Autodesk Inventor part; units mm, degrees
ref_plane "YZ Plane" through (0, 0, 0) normal (1, 0, 0) x (0, 1, 0)
ref_plane "XZ Plane" through (0, 0, 0) normal (0, 1, 0) x (-1, 0, 0)
ref_plane "XY Plane" through (0, 0, 0) normal (0, 0, 1) x (1, 0, 0)
sketch "Sketch1" plane through (0, 0, 0) normal (1, 0, 0) x (0, 1, 0)
  circle A0 centre (0, 0) radius 2.25
  circle A1 centre (0, 0) radius 4.75
  line L0 (0, 4.75) -> (-10.16, 4.75)
  line L1 (0, -4.75) -> (-10.16, -4.75)
  line L2 (-10.16, 4.75) -> (-10.16, -4.75)
  dimension "d0" = 4.5
  dimension "d1" = 9.5
  dimension "d2" = 10.16
  dimension "d3" = 10.16
extrude "Extrusion1" add sketch "Sketch1" along normal blind 7.62
ref_plane "Work Plane1" through (15.24, 0, 0) normal (1, 0, 0) x (0, 0, -1)
mirror "Mirror1" about plane through (15.24, 0, 0) normal (1, 0, 0) of "Extrusion1"
sketch "Sketch2" plane through (30.48, -10.16, 4.75) normal (1, 0, 0) x (0, 0, -1)
  circle A0 centre (4.75, 10.16) radius 2.25
  line L0 (7.5, 8.5723) -> (4.75, 6.9846)
  line L1 (4.75, 6.9846) -> (2, 8.5723)
  line L2 (2, 8.5723) -> (2, 11.7477)
  line L3 (2, 11.7477) -> (4.75, 13.3354)
  line L4 (4.75, 13.3354) -> (7.5, 11.7477)
  line L5 (7.5, 11.7477) -> (7.5, 8.5723)
  dimension "d7" = 5.5
extrude "Extrusion2" cut sketch "Sketch2" against normal blind 1.5
sketch "Sketch3" plane through (0, 0, 0) normal (-1, 0, 0) x (0, 0, 1)
  circle A0 centre (0, 0) radius 2.75
  dimension "d10" = 5.5
extrude "Extrusion3" cut sketch "Sketch3" against normal blind 1.5
sketch "Sketch4" plane through (0, 0, 0) normal (-1, 0, 0) x (0, 0, 1)
  line L0 (4.75, 0) -> (7.925, -10.16)
  line L1 (4.75, -10.16) -> (-4.75, -10.16)
  line L2 (7.925, -10.16) -> (4.75, -10.16)
  line L3 (4.75, 0) -> (4.75, -10.16)
  point P0 (0, 0)
  dimension "d13" = 3.175
extrude "Extrusion4" add sketch "Sketch4" against normal up to surface (30.48 mm away)
sketch "Sketch5" plane through (0, 0, 0) normal (-1, 0, 0) x (0, 0, 1)
  line L0 (-4.75, -10.16) -> (-4.75, 0)
  line L1 (-4.75, -10.16) -> (-4.75, -31.75)
  line L2 (4.75, 0) -> (4.75, -10.16)
  line L3 (7.925, -10.16) -> (14.6719, -31.75)
  line L4 (4.75, 0) -> (7.925, -10.16)
  line L5 (-4.75, -31.75) -> (14.6719, -31.75)
  line L6 (7.925, -10.16) -> (-4.75, -10.16)
  line L7 (-4.75, -10.16) -> (7.925, -10.16)
  point P0 (0, 0)
  dimension "d16" = 31.75
extrude "Extrusion5" add sketch "Sketch5" against normal up to surface (30.48 mm away) contours L6 L3 L5 L1
sketch "Sketch6" plane through (7.62, 0, -4.75) normal (0, 0, -1) x (-1, 0, 0)
  line L0 (-22.86, -31.75) -> (-22.86, 0)
  line L1 (-22.86, -6.35) -> (-16.0541, -31.75)
  line L2 (7.62, -31.75) -> (-22.86, -31.75)
  line L3 (7.62, -6.35) -> (0.8141, -31.75)
  line L4 (7.62, 0) -> (7.62, -31.75)
  line L5 (-22.86, -6.35) -> (-22.86, -31.75)
  line L6 (-22.86, -31.75) -> (-16.0541, -31.75)
  line L7 (0.8141, -31.75) -> (7.62, -31.75)
  line L8 (7.62, -6.35) -> (7.62, -31.75)
  dimension "d20" = 15
  dimension "d21" = 6.35
  dimension "d22" = 15
  dimension "d23" = 6.35
extrude "Extrusion6" cut sketch "Sketch6" against normal through all
sketch "Sketch7" plane through (6.8059, -31.75, 14.6719) normal (0, -1, 0) x (1, 0, 0)
  line L0 (16.0541, -12.4219) -> (16.0541, -16.9219)
  line L1 (16.0541, -19.4219) -> (16.0541, -9.9219)
  line L2 (16.0541, -9.9219) -> (16.0541, -19.4219)
  line L3 (0.8141, -12.4219) -> (0.8141, -16.9219)
  line L4 (0.8141, -9.9219) -> (0.8141, -19.4219)
  line L5 (0.8141, -19.4219) -> (0.8141, -9.9219)
  line L6 (0.8141, -19.4219) -> (0.8141, -9.9219)
  line L7 (0, 0) -> (16.8682, 0)
  line L8 (5.8941, 0) -> (10.9741, 0)
  line L9 (10.9741, 0) -> (10.9741, -9.9219)
  line L10 (10.9741, -9.9219) -> (5.8941, -9.9219)
  line L11 (5.8941, -9.9219) -> (5.8941, 0)
  line L12 (5.8941, -9.9219) -> (-12.9487, -9.9219)
  line L13 (-12.9487, -9.9219) -> (-12.9487, 3.2333)
  line L14 (-12.9487, 3.2333) -> (5.8941, 3.2333)
  line L15 (5.8941, 3.2333) -> (5.8941, -9.9219)
  line L16 (10.9741, -9.9219) -> (26.322, -9.9219)
  line L17 (26.322, -9.9219) -> (26.322, 1.6077)
  line L18 (26.322, 1.6077) -> (10.9741, 1.6077)
  line L19 (10.9741, 1.6077) -> (10.9741, -9.9219)
  point P0 (-6.8059, -14.6719)
  dimension "d28" = 5.08
  dimension "d29" = 0
  dimension "d30" = 5.8941
  dimension "d31" = 5.8941
extrude "Extrusion7" cut sketch "Sketch7" against normal through all contours L11 L12 L13 L14 L15 | L19 L18 L17 L16 L9
sketch "Sketch8" plane through (17.78, -31.75, 14.6719) normal (1, 0, 0) x (0, 0, -1)
  line L0 (9.9219, 21.59) -> (19.4219, 21.59)
  line L1 (9.9219, 21.59) -> (19.4219, 21.59)
  line L2 (9.9219, 21.59) -> (5.1304, 21.59)
  line L3 (5.1304, 21.59) -> (9.9219, 31.75)
  line L4 (9.9219, 31.75) -> (9.9219, 21.59)
  line L5 (9.9219, 0) -> (9.9219, 25.4)
  point P0 (14.6719, 31.75)
extrude "Extrusion8" cut sketch "Sketch8" against normal up to surface (5.08 mm away)
equation "\"d30\" = d31"
properties part number "Camera Holder"
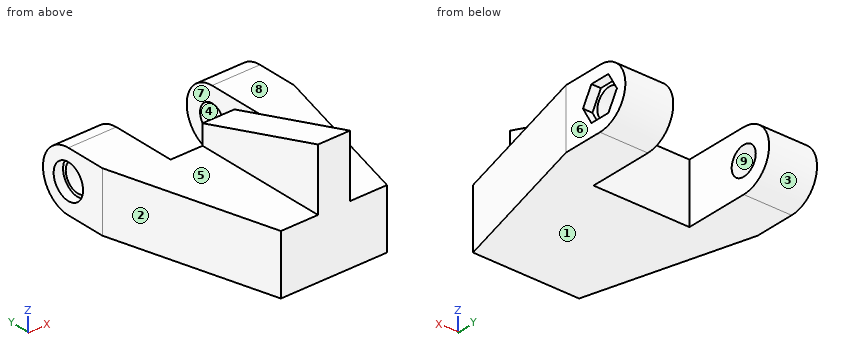
Input: part model. Units: mm. Frame: model coordinates. Face numbers are marked on the shaded views. A direction names the side the tool comes from. Round coordinates to 2 decimals unless told otherwise and drop trailing zeros. Loops run counter-clockwise (first coordinate to the right, second up) from the corner with the lowest first, then second, coordinate; pieces in that order, holes last. Notation, with made-up numbers: M 52.25,22 L 67.25,22 A10 cw 67.25,41 Z; hole C 88,59 d5. An arc over 180 degrees is marked long. Answer in a Markdown table with one row per item. Add a question column.
1. Ray query, probe 1 along Z at (x, y) = (4, 0); probe 2 along X at (y, z) = (-1, -2.5); probe 3 along Y at (x, z) = (13.5, -1.75). Return the intervals inside material, ascending.
2. Set-up query: the marked faces 5, 6, 7, 8 and 9. Return all of +Z, -Z, +X, -X, +Y, -Y with unobstructed straight access to the full face (end or side cutting, diameter ignored); none if empty.
3. Section A-A (y = -7). Output: boundary loops of the cut face in (x, z), and give its area (3 significant figures).
4. Section D-D (y = -13). Output: boundary loops of the cut face in (x, z).
5. Contact query for flat-ended pins moving along their axis: pin 1 (6.5 mm diameter, centred on x = 22.5, y = -20, fed in from +Z); pin 2 (10 mm diameter, centred on y = -15.5, z = 7, fed in from -X); pin 3 (4 mm diameter, centred on x = 14, z = 0, fed in from +Y); pin 4 (1.6 mm diameter, centred on y = -0.5, z = -0.5, fed in from +X). Output: stop coordinate, or through.
6. Section B-B (z = 6.25). Output: boundary loops of the cut face in (x, y).
7. Section C-C (x = 9). Output: boundary loops of the cut face in (y, z), and give its area (3 significant figures).
8. Mould query, pull axis Y, two halves, no side actions, for the marked faces 1, 2, 3 and 4. Classes: released by +Y, released by -Y, zero draft, split by the parting line, or undercut.
Values follow:
| question | item | result |
|---|---|---|
| 1 | probe 1 | -4.75 to -2.25, 2.25 to 4.75 |
| 1 | probe 2 | 1.5 to 7.62, 22.86 to 28.98 |
| 1 | probe 3 | -31.75 to -10.16 |
| 2 | face 5 | +Z, -X, +Y, -Y |
| 2 | face 6 | +Z, -Z, +X, +Y, -Y |
| 2 | face 7 | +Z, -Z, +Y |
| 2 | face 8 | +Z, +X, +Y, -Y |
| 2 | face 9 | +X, -X |
| 3 | outline | M 0.17,-4.75 L 7.62,-4.75 L 7.62,4.75 L 0.17,4.75 Z; M 22.86,-4.75 L 30.31,-4.75 L 30.31,4.75 L 22.86,4.75 Z |
| 3 | area | 141 mm^2 |
| 4 | outline | M 1.78,-4.75 L 28.7,-4.75 L 28.7,4.75 L 17.78,4.75 L 17.78,8.81 L 12.7,8.81 L 12.7,4.75 L 1.78,4.75 Z |
| 5 | pin 1 | z = 4.75 |
| 5 | pin 2 | x = 1.26 |
| 5 | pin 3 | y = -10.16 |
| 5 | pin 4 | through |
| 6 | outline | M 12.7,-31.75 L 17.78,-31.75 L 17.78,-10.16 L 12.7,-10.16 Z |
| 7 | outline | M -31.75,-4.75 L -10.16,-4.75 L -10.16,4.75 L -31.75,4.75 Z |
| 7 | area | 205 mm^2 |
| 8 | face 1 | zero draft |
| 8 | face 2 | released by -Y |
| 8 | face 3 | released by +Y |
| 8 | face 4 | undercut |
